from build123d import *

# Parameters (mm, degrees)
BOSS_EXTRUDE1_DEPTH     = 44.9
FILLET1_R               = 2.1
BOSS_EXTRUDE2_DEPTH     = 2
CUT_EXTRUDE1_DEPTH      = 61.269699517
CUT_EXTRUDE1_DEPTH_BACK = 61.269699517
FILLET2_R               = 1


with BuildPart() as part:
    # Sketch1 → Boss-Extrude1 (new body)
    with BuildSketch(Plane.XY):
        with BuildLine():
            Line((-11.688749537, -31.975), (-19.771653306, -17.975))
            ThreePointArc((-19.771653306, -17.975), (-19.771653306, -6.025), (-9.422649731, -0.05))
            Line((-9.422649731, -0.05), (9.422649731, -0.05))
            ThreePointArc((9.422649731, -0.05), (19.771653306, -6.025), (19.771653306, -17.975))
            Line((19.771653306, -17.975), (11.688749537, -31.975))
            Line((11.688749537, -31.975), (-11.688749537, -31.975))
        make_face()
    extrude(amount=-BOSS_EXTRUDE1_DEPTH)

    # Fillet1
    fillet1_edges = [part.edges().sort_by_distance(p)[0] for p in [
        (15.730201422, -24.975, -44.9),
        (19.771653306, -6.025, -44.9),
        (0, -0.05, -44.9),
        (-19.771653306, -6.025, -44.9),
        (-15.730201422, -24.975, -44.9),
    ]]
    fillet(fillet1_edges, radius=FILLET1_R)

    # Sketch2 → Boss-Extrude2 (add)
    with BuildSketch(Plane.XY):
        with BuildLine():
            Line((15.152851153, -31.975), (22.369729517, -19.475))
            ThreePointArc((22.369729517, -19.475), (22.369729517, -4.525), (9.422649731, 2.95))
            Line((9.422649731, 2.95), (-9.422649731, 2.95))
            ThreePointArc((-9.422649731, 2.95), (-22.369729517, -4.525), (-22.369729517, -19.475))
            Line((-22.369729517, -19.475), (-15.152851153, -31.975))
            Line((-15.152851153, -31.975), (15.152851153, -31.975))
        make_face()
    extrude(amount=BOSS_EXTRUDE2_DEPTH)

    # Sketch3 → Cut-Extrude1 (cut, two sides: drawn at the far end of the back side and taken through both)
    with BuildSketch(Plane.XY.offset(-CUT_EXTRUDE1_DEPTH_BACK)):
        with BuildLine():
            Line((-3.447387849, -1.05), (3.447387849, -1.05))
            ThreePointArc((3.447387849, -1.05), (4.861601412, -1.635786438), (5.447387849, -3.05))
            Line((5.447387849, -3.05), (5.447387849, -5.05))
            Line((5.447387849, -5.05), (5.10836082, -5.981469107))
            ThreePointArc((5.10836082, -5.981469107), (1.679610771, -18.777738497), (0.525, -31.975))
            Line((0.525, -31.975), (-0.525, -31.975))
            ThreePointArc((-0.525, -31.975), (-1.679610771, -18.777738497), (-5.10836082, -5.981469107))
            Line((-5.10836082, -5.981469107), (-5.447387849, -5.05))
            Line((-5.447387849, -5.05), (-5.447387849, -3.05))
            ThreePointArc((-5.447387849, -3.05), (-4.861601412, -1.635786438), (-3.447387849, -1.05))
        make_face()
    extrude(amount=CUT_EXTRUDE1_DEPTH + CUT_EXTRUDE1_DEPTH_BACK, mode=Mode.SUBTRACT)

    # Fillet2
    fillet2_edges = [part.edges().sort_by_distance(p)[0] for p in [
        (-0.525, -31.975, -21.45),
        (0.525, -31.975, -21.45),
    ]]
    fillet(fillet2_edges, radius=FILLET2_R)


solid = part.part
For this review, take the finished solid that the model builds, in its own axes (mm). A direction names the side the tool comes from. Round coordinates to 2 decimals unless told otherwise and drop trailing zeros. Loops run counter-clockwise (first coordinate to the right, second up) from the corner with the lowest first, then second, coordinate; pieces in that order, holes last. Notation, with made-up numbers: (-31, -27.5) - (23, -27.5) arc R34 cw to (23, 11.5) - close; hole circle Ø2 at (60.5, 63.5). An arc over 180 degrees is marked (long way). Put each result on its own line as item: value. Start each with the question number.
1. Consider section A-A on z = -16.5. State the section outline as (x, y) points (3 decimals).
2. Insertion check: P1, Ø1.5, axis at x = 5, z = -8.5, coming from the +Y side; P2, Ø0.6, axis at y = -4, z = -21.5, coming from the +X side; P3, Ø1, axis at y = -15, z = -32.5, coming from the -X side. Each pin has a flat end and moves straight along its axis. Give the tip position at first contact, or say it passes through.
3. Consider section B-B on x = -2.5. State the section outline as (y, z) points (3 decimals).
4. Consider section C-C on x = -8.5. State the section outline as (y, z) points (3 decimals), plus the area to 3 significant figures.
5. For probe 1 along X at (y, z) = (-25.5, -24); probe 2 along Z at (x, y) = (15, -22.5); probe 3 along Z at (x, y) = (20, -1.5), list the stretches that pass through material, from the lowest coordinate up. Write a range as [from, to].
6. Mouldability with a two-part tool opening along Y and no side actions: class faces 1 (the cylindrical face through (0.13, -0.42, -43.99)), 2 (the flat face through (7, -31.975, -22)), 3 (the flat face through (0, -1.05, -22)) as +Y half, -Y half, draft (parallel to the pull), parting line (faces both ways), or undercut.
7. For faces 4 (the flat face through (5.447, -4, -22)), 5 (the flat face through (0, -0.05, -21)), 6 (the cylindrical face through (19.7, -5.9, -21.1)), list the 3-axis set-ups (+Z, -Z, +X, -X, +Y, -Y) from which the entire face can be reached by the end or side of a thin tool; tool diameter is ignored.
Result sheet:
1. outline: (-19.772, -17.975) - (-11.689, -31.975) - (-1.532, -31.975) arc R1 ccw to (-0.532, -30.962) arc R76 ccw to (-5.108, -5.981) - (-5.447, -5.05) - (-5.447, -3.05) arc R2 cw to (-3.447, -1.05) - (3.447, -1.05) arc R2 cw to (5.447, -3.05) - (5.447, -5.05) - (5.108, -5.981) arc R76 ccw to (0.532, -30.962) arc R1 ccw to (1.532, -31.975) - (11.689, -31.975) - (19.772, -17.975) arc R11.95 ccw to (9.423, -0.05) - (-9.423, -0.05) arc R11.95 ccw to start
2. P1: y = -0.05
2. P2: x = 18.56
2. P3: x = -21.11
3. outline: (-31.975, -44.9) - (-14.762, -44.9) - (-14.762, 2) - (-31.975, 2) - close; (-1.05, -44.589) arc R2.1 ccw to (-0.05, -42.8) - (-0.05, 0) - (2.95, 0) - (2.95, 2) - (-1.05, 2) - close
4. outline: (-31.975, -44.9) - (-2.15, -44.9) arc R2.1 ccw to (-0.05, -42.8) - (-0.05, 0) - (2.95, 0) - (2.95, 2) - (-31.975, 2) - close
4. area: 1,500 mm^2
5. probe 1: [-15.43, -0.8], [0.8, 15.43]
5. probe 2: [-44.89, 2]
5. probe 3: [0, 2]
6. face 1: +Y half
6. face 2: -Y half
6. face 3: undercut
7. face 4: +Z, -Z
7. face 5: -Z, +X, -X, +Y
7. face 6: -Z, +X
